```python
from build123d import *

# Parameters (mm, degrees)
SKETCH1_R               = 2.1
BOSS_EXTRUDE1_DEPTH     = 3
BOSS_EXTRUDE2_DEPTH     = 40
FILLET1_R               = 18
SKETCH2_W               = 80
SKETCH2_H               = 3
BOSS_EXTRUDE3_DEPTH     = 8
FILLET2_R               = 2
CUT_EXTRUDE1_DEPTH      = 111.696432989
CUT_EXTRUDE1_DEPTH_BACK = 111.696432989
SKETCH3_R               = 1.6
FILLET3_R               = 3


# Some blends are built 0.0001 mm under size
with BuildPart() as part:
    # Sketch1 → Boss-Extrude1 (new body)
    with BuildSketch(Plane.XY):
        with BuildLine():
            Line((0, 11.023468057), (95, 11.023468057))
            ThreePointArc((95, 11.023468057), (106.023468057, 0), (95, -11.023468057))
            Line((95, -11.023468057), (0, -11.023468057))
            ThreePointArc((0, -11.023468057), (-11.023468057, 0), (0, 11.023468057))
        make_face()
        Circle(SKETCH1_R, mode=Mode.SUBTRACT)
        with Locations((95, 0)):
            Circle(SKETCH1_R, mode=Mode.SUBTRACT)
    extrude(amount=BOSS_EXTRUDE1_DEPTH)

    # 3DSketch1 → Boss-Extrude2 (add, symmetric)
    with BuildSketch(Plane(origin=(47.5, 3.976531943, 0), x_dir=(0, -0.9805806756909202, -0.19611613513818404), z_dir=(-1, 0, 0))):
        Polygon((0, 0), (0.980580676, -4.902903378), (25.495097568, 0), (24.514516892, 4.902903378), align=None)
    extrude(amount=BOSS_EXTRUDE2_DEPTH, both=True)

    # Fillet1
    # the kernel refuses this fillet: 18 mm, written as the material it takes off along each edge
    with BuildSketch(Plane(origin=(118.624748995, 3.976531943, -5), x_dir=(0, 0, 1), z_dir=(-1, 0, 0))) as fillet1_piece_1:
        with BuildLine():
            CenterArc((18, -12.449899598), FILLET1_R, 136.238257307, 43.761742693)
            Line((0, -12.449899598), (-0.36, -12.449899598))
            Line((-0.36, -12.449899598), (-0.36, 0))
            Line((-0.36, 0), (0, 0.36))
            ThreePointArc((0, 0.36), (2.5, 0.36), (4.74, 0.248997992))
            Line((4.74, 0.248997992), (5, 0))
        make_face()
    extrude(amount=142.24949799, mode=Mode.SUBTRACT)

    # Sketch2 → Boss-Extrude3 (add)
    with BuildSketch(Plane(origin=(0, 0, -5), x_dir=(-1, 0, 0), z_dir=(0, 0, -1))):
        with Locations((-47.5, -19.523468057)):
            Rectangle(SKETCH2_W, SKETCH2_H)
    extrude(amount=BOSS_EXTRUDE3_DEPTH)

    # Fillet2
    fillet2_edges = [part.edges().sort_by_distance(p)[0] for p in [
        (47.5, -18.023468057, -5),
    ]]
    fillet(fillet2_edges, radius=FILLET2_R)

    # Sketch3 → Cut-Extrude1 (cut, two sides: drawn at the far end of the back side and taken through both)
    with BuildSketch(Plane(origin=(0, -18.023468057, 0), x_dir=(1, 0, 0), z_dir=(0, 1, 0)).offset(-CUT_EXTRUDE1_DEPTH_BACK)):
        with Locations(Location((17.5, 10.125300862, 0), (0, 0, 90))):
            Circle(SKETCH3_R)
        with Locations(Location((77.5, 10.125300862, 0), (0, 0, 90))):
            Circle(SKETCH3_R)
    extrude(amount=CUT_EXTRUDE1_DEPTH + CUT_EXTRUDE1_DEPTH_BACK, mode=Mode.SUBTRACT)

    # Fillet3
    fillet3_edges = [part.edges().sort_by_distance(p)[0] for p in [
        (7.5, -1.765163723, -3.703293088),
        (87.5, -1.765163723, -3.703293088),
        (7.5, -18.023468057, -10),
        (7.5, -17.43768162, -5.585786438),
        (87.5, -17.43768162, -5.585786438),
        (87.5, -18.023468057, -10),
        (87.5, -12.248417856, -5),
        (7.5, -12.248417856, -5),
    ]]
    fillet(fillet3_edges, radius=FILLET3_R - 0.0001)  # a hair under: the kernel refuses the full size


solid = part.part
```
Model file for the job. Use its own axes, mm. A direction names the side the tool comes from. Coordinates: 2 decimals unless noted, no trailing zeros. Loops run counter-clockwise (first coordinate to the right, second up) from the corner with the lowest first, then second, coordinate; pieces in that order, holes last. Notation, with made-up numbers: (87.25, 30) - (135.25, 30) arc R8 cw to (135.25, 42) - close; hole circle Ø6 at (77.25, 82.25). An arc over 180 degrees is marked (long way). Answer as a JSON object with one key per item and string values. Group by question number.
(1) Cut at A-A (x = 17.5). Give the cut face in (y, z).
(2) Two-plate mould, pull along Z, no slides. Class faces 6 (the face through (48, -11.023, 1)), 7 (the face through (48.02, -1.68, -3.67)), 8 (the face through (75.914, -19.544, -9.917)), 9 (the face through (47, -16, 0)): released by +Z, released by -Z, zero draft, split by the parting line, or undercut.
(3) Tool access for faces 1 (the face through (48, -18.023, -10)), 2 (the face through (15.914, -19.544, -9.917)), 3 (the face through (8.4, -18.88, -9.96)), 4 (the face through (86.645, -18.926, -9.958)), 5 (the face through (87.5, -13, -1)): list every direction of +Z, -Z, +X, -X, +Y, -Y with a clear straight run to the whole face (end or side of a thin tool).
(4) Probe line 1 along Z through (x, y) = (77.5, -18.9); line 2 along Y through (x, z) = (51, 1.25); line 3 along Z through (x, y) = (84.5, -19). List the from-to ranges inside material, lowest first.
(5) Flat gauge pins, fed straight in: pin 1 (1 mm diameter, centred on x = 71.5, y = -14.5, fed in from +Z); pin 2 (1.5 mm diameter, centred on x = 63.5, z = 2, fed in from -Y); pin 3 (1 mm diameter, centred on x = 86.5, y = 7, fed in from -Z); pin 4 (3 mm diameter, centred on x = 17.5, z = -10.13, fed in from -Y). Where does each tip first touch, or does it go through?
(6) Cut at D-D (y = 0). State how many separate pieces and enclosed holes the cut face has, then the cut area to 3 significant figures.
(7) Cut at C-C (x = 37.5). Give the cut face in (y, z).
(8) Cut at B-B (z = 1.25). Give the cut face in (x, y), then the cut area to 3 significant figures.
Geometry says:
{
 "1": {"outline": "(-21.02, -13) - (-18.02, -13) - (-18.02, -11.73) - (-21.02, -11.73) - close; (-21.02, -8.53) - (-18.02, -8.53) - (-18.02, -7) arc R2 cw to (-16.02, -5) - (-8.47, -5) arc R18 ccw to (3.98, 0) - (11.02, 0) - (11.02, 3) - (-11.02, 3) - (-11.02, 0) - (-21.02, 0) - close"},
 "2": {"face 6": "zero draft", "face 7": "released by -Z", "face 8": "undercut", "face 9": "released by +Z"},
 "3": {"face 1": "-Z, +X, -X, +Y", "face 2": "+Y, -Y", "face 3": "-Z, -X, +Y", "face 4": "-Z, +X, +Y", "face 5": "-Z, +X, +Y, -Y"},
 "4": {"line 1": "z = -13 to -11.73, -8.53 to 0", "line 2": "y = -11.02 to 11.02", "line 3": "z = -13 to 0"},
 "5": {"pin 1": "stops at z = 0", "pin 2": "stops at y = -11.02", "pin 3": "stops at z = 0", "pin 4": "passes through"},
 "6": {"separate pieces": "3", "enclosed holes": "0", "area": "552 mm^2"},
 "7": {"outline": "(-21.02, -13) - (-18.02, -13) - (-18.02, -7) arc R2 cw to (-16.02, -5) - (-8.47, -5) arc R18 ccw to (3.98, 0) - (11.02, 0) - (11.02, 3) - (-11.02, 3) - (-11.02, 0) - (-21.02, 0) - close"},
 "8": {"outline": "(0, -11.02) - (95, -11.02) arc R11.02 ccw to (95, 11.02) - (0, 11.02) arc R11.02 ccw to start; hole circle Ø4.2 at (0, 0); hole circle Ø4.2 at (95, 0)", "area": "2,450 mm^2"}
}
